Here's how the part is built. I have some questions about the finished solid (model axes, mm). Face numbers are marked on the shaded views. A direction names the side the tool comes from. Give positions to 0.01 mm unless a question says otherwise; leave off trailing zeros. Order: outer loops, then holes, each group sorted by start corner. A loop starts at its lowest first (then second) coordinate and runs counter-clockwise, first axis right, second up. Notation, with made-up numbers: M 78,55 L 127,55 A16 ccw 127,83 Z; hole C -20,31 d9. An arc over 180 degrees is marked long. Use one line per item in the form item = value.
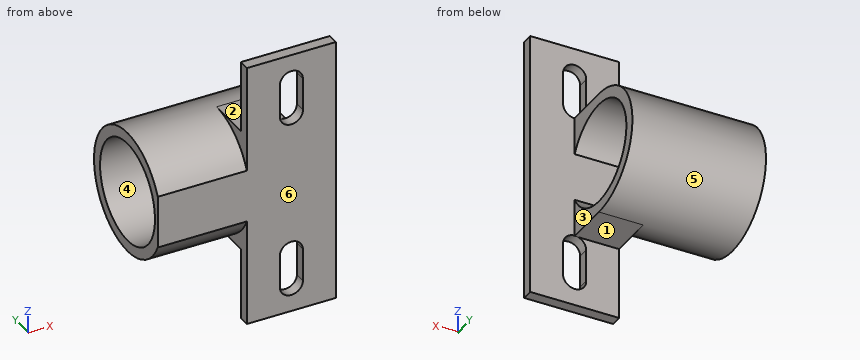
Autodesk Inventor part; units mm, degrees
ref_plane "Work Plane2" through (3.4844, 0, -27.9715) normal (0, 0, 1) x (1, 0, 0)
ref_plane "YZ Plane" through (0, 0, 0) normal (1, 0, 0) x (0, 1, 0)
ref_plane "XZ Plane" through (0, 0, 0) normal (0, 1, 0) x (-1, 0, 0)
sketch "Sketch1" plane through (0, 0, 0) normal (0, 1, 0) x (-1, 0, 0)
  line L0 (-3.4844, 10.1285) -> (-28.8844, 10.1285)
  line L1 (-28.8844, 10.1285) -> (-28.8844, -66.0715)
  line L2 (-28.8844, -66.0715) -> (-3.4844, -66.0715)
  line L3 (-3.4844, -66.0715) -> (-3.4844, 10.1285)
  dimension "d0" = 25.4
  dimension "d1" = 76.2
extrude "Extrusion1" add sketch "Sketch1" against normal blind 3.175
sketch "Sketch7" plane through (3.4844, 0, -66.0715) normal (-1, 0, 0) x (0, 0, 1)
  line L0 (76.2, -3.175) -> (0, -3.175)
  circle A0 centre (38.1, 12.7254) radius 6.35
  circle A1 centre (38.1, 12.7254) radius 14.4272
  arc A2 (45.6508, -3.175) -> (30.5492, -3.175) centre (38.1, 12.7254) ccw
  point P0 (38.1, -3.175)
  dimension "d24" = 15.9004
  dimension "d25" = 12.7
  dimension "d26" = 28.8544
  dimension "d57" = 3.175
extrude "Extrusion7" add sketch "Sketch7" along normal mid plane 25.4 contours L0 A2
sketch "Sketch8" plane through (16.1844, 0, -66.0715) normal (1, 0, 0) x (0, 0, -1)
  line L0 (-25.9385, 0) -> (-31.3023, 0)
  arc A0 (-25.9385, 0) -> (-50.2615, 0) centre (-38.1, 12.7254) ccw
  arc A1 (-30.5492, -3.175) -> (-45.6508, -3.175) centre (-38.1, 12.7254) ccw
  line L1 (-55.7022, 12.7254) -> (-55.7022, 0)
  line L2 (-50.2615, 0) -> (-76.2, 0)
  line L3 (-20.4978, 12.7254) -> (-20.4978, 0)
  line L4 (-76.2, 0) -> (0, 0)
extrude "Extrusion8" add sketch "Sketch8" against normal blind 12.7 contours A0 L3 L4 | L2 L1 A0
sketch "Sketch10" plane through (0, 0, 0) normal (0, 1, 0) x (1, 0, 0)
  arc A0 (12.8824, -2.064) -> (19.4864, -2.064) centre (16.1844, -2.064) ccw
  arc A1 (19.4864, 7.207) -> (12.8824, 7.207) centre (16.1844, 7.207) ccw
  line L0 (12.8824, 7.207) -> (12.8824, -2.064)
  line L1 (19.4864, 7.207) -> (19.4864, -2.064)
  line L2 (19.4864, 2.5715) -> (20.5922, 2.5715)
  line L3 (29.0114, 27.9715) -> (23.9538, 27.9715)
  line L4 (16.1844, 10.509) -> (16.1844, -5.366)
  line L5 (28.8844, 66.0715) -> (3.4844, 66.0715)
  line L6 (28.8844, -10.1285) -> (28.8844, 66.0715)
  dimension "d43" = 6.604
  dimension "d44" = 6.604
  dimension "d45" = 25.4
  dimension "d53" = 15.875
extrude "Extrusion10" cut sketch "Sketch10" against normal blind 25.4
sketch "Sketch11" plane through (-9.2156, 0, -66.0715) normal (-1, 0, 0) x (0, 0, 1)
  circle A0 centre (38.1, 12.7254) radius 14.4272
  arc A1 (45.6508, -3.175) -> (30.5492, -3.175) centre (38.1, 12.7254) ccw
  line L0 (30.5492, -3.175) -> (45.6508, -3.175)
extrude "Extrusion11" add sketch "Sketch11" along normal blind 12.7
ref_plane "Work Plane2" through (3.4844, 0, -27.9715) normal (0, 0, 1) x (1, 0, 0)
mirror "Mirror1" about plane through (3.4844, 0, -27.9715) normal (0, 0, 1) of "Extrusion10"
properties part number "Bearing mount"
Q1. Thinking about a two-plate mould opening in Y: for the marked faces 4, 5 and 6, which applies, +Y half, -Y half, draft (parallel to the pull), parting line (faces both ways), or undercut?
Found:
face_4 = undercut
face_5 = parting line
face_6 = -Y half
Q2. I want a section at B-B on y = 10. Write out the boundary of the cut face in (x, z).
Found:
outline = M -21.92,-45.36 L 3.48,-45.36 L 3.48,-45.57 L 16.18,-45.57 L 16.18,-42.14 L -21.92,-42.14 Z; M -21.92,-13.8 L 16.18,-13.8 L 16.18,-10.37 L 3.48,-10.37 L 3.48,-10.58 L -21.92,-10.58 Z
Q3. On a 3-axis mill with a long thin cutter (end or side, diameter ignored), from which of +Z, -Z, +X, -X, +Y, -Y can I reach the whole of each face in a straight line? I mean the marked faces 1, 2 and 3. Say none if no direction works.
Found:
face_1 = -Z, +X, -X, +Y
face_2 = +Z, +X, -X, +Y
face_3 = +Z, -Z, +X, +Y
Q4. I need wall thicknesses on L1, parallel to X at y = 4, z = -39.5; L2, parallel to Y at x = 26.5, z = -50.5 (3 decimals); L3, parallel to Z at x = -13, y = 8. Which ranges of each line are inside material? Lowest first, please.
Found:
L1 = -21.92 to 16.18
L2 = -3.175 to 0
L3 = -44.93 to -41.6, -14.34 to -11.02
Q5. I want a section at D-D on z = -60.5. Write out the boundary of the cut face in (x, y) (3 decimals), then the cut area to 3 significant figures.
Found:
outline = M 3.484,-3.175 L 14.019,-3.175 L 14.019,0 L 3.484,0 Z; M 18.35,-3.175 L 28.884,-3.175 L 28.884,0 L 18.35,0 Z
area = 66.9 mm²
Q6. I'm going to push flat-ended pins straight in: pin 1 Ø3.5 at (y, z) = (-2, -3) entering from -X; pin 2 Ø4 at (x, y) = (7, 5) entering from +Z; pin 3 Ø14 at (x, y) = (11.5, 8.5) entering from -Z. Where does each tip first touch, or does it pass through?
Found:
pin_1 = 3.48
pin_2 = -10.37
pin_3 = -45.57
Q7. I want a section at C-C on x = 14. Write out the boundary of the cut face in (y, z) (1 decimal).
Found:
outline = M -3.2,-66.1 L 0,-66.1 L 0,-60.5 L -3.2,-60.5 Z; M -3.2,-46.3 L 0,-46.3 L 0,-45.6 L 12.7,-45.6 A17.6 ccw 12.7,-10.4 L 0,-10.4 L 0,-9.7 L -3.2,-9.7 Z; M -3.2,4.5 L 0,4.5 L 0,10.1 L -3.2,10.1 Z; hole M 0,-34.8 A14.4 ccw long 0,-21.2 Z
Q8. I want a section at A-A on z = -5.5. Write out the boundary of the cut face in (x, y) (3 decimals).
Found:
outline = M 3.484,-3.175 L 12.882,-3.175 L 12.882,0 L 3.484,0 Z; M 19.486,-3.175 L 28.884,-3.175 L 28.884,0 L 19.486,0 Z
